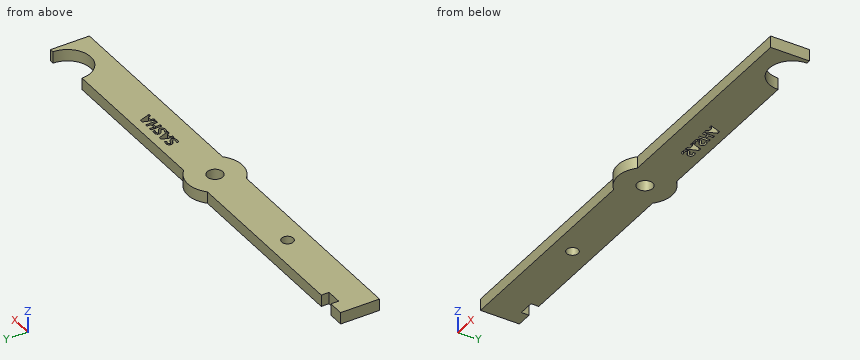
from build123d import *

# Parameters (mm, degrees)
F0_R     = 1.5
F0_R_2   = 2
F1_DEPTH = 3


with BuildPart() as f1:
    # F0 (on Top) → F1 (new body)
    with BuildSketch(Plane.XY):
        with BuildLine():
            Line((-56, 5), (-60, 5))
            Line((-60, 5), (-60, -5))
            Line((-60, -5), (-4.8989794856, -5))
            ThreePointArc((-4.8989794856, -5), (-7, 0), (-4.8989794856, 5))
            Line((-4.8989794856, 5), (-52, 5))
            Line((-52, 5), (-52, 3))
            Line((-52, 3), (-56, 3))
            Line((-56, 3), (-56, 5))
        make_face()
        with Locations((-30, 0)):
            Circle(F0_R, mode=Mode.SUBTRACT)
        with BuildLine():
            ThreePointArc((7, 0), (6.4534043883, -2.7117470016), (4.8989794856, -5))
            Line((4.8989794856, -5), (60, -5))
            Line((60, -5), (60, 5))
            Line((60, 5), (59, 5))
            ThreePointArc((59, 5), (53, -1), (47, 5))
            Line((47, 5), (4.8989794856, 5))
            ThreePointArc((4.8989794856, 5), (6.4534043883, 2.7117470016), (7, 0))
        make_face()
        with BuildLine():
            add(Edge.make_bspline(
                [(16.4754206125, 1.2379939809), (16.6207250703, 1.049862946), (16.6207250703, 0.7763846611)],
                knots=[0, 0, 0, 1, 1, 1], degree=2))
            add(Edge.make_bspline(
                [(16.6207250703, 0.7763846611), (16.6207250703, 0.3976753583), (16.3481644978, 0.1795657195)],
                knots=[0, 0, 0, 1, 1, 1], degree=2))
            add(Edge.make_bspline(
                [(16.3481644978, 0.1795657195), (16.0756039253, -0.0385439193), (15.5904399881, -0.0385439193)],
                knots=[0, 0, 0, 1, 1, 1], degree=2))
            add(Edge.make_bspline(
                [(15.5904399881, -0.0385439193), (15.1425963539, -0.0385439193), (14.798760121, 0.1303151559)],
                knots=[0, 0, 0, 1, 1, 1], degree=2))
            Line((14.798760121, 0.1303151559), (14.798760121, 0.6809425751))
            add(Edge.make_bspline(
                [(14.798760121, 0.6809425751), (15.0814155295, 0.5542982687), (15.2775000716, 0.5029063762)],
                knots=[0, 0, 0, 1, 1, 1], degree=2))
            add(Edge.make_bspline(
                [(15.2775000716, 0.5029063762), (15.4735846136, 0.4515144838), (15.6363256064, 0.4515144838)],
                knots=[0, 0, 0, 1, 1, 1], degree=2))
            add(Edge.make_bspline(
                [(15.6363256064, 0.4515144838), (15.8308806279, 0.4515144838), (15.9351939334, 0.5258491854)],
                knots=[0, 0, 0, 1, 1, 1], degree=2))
            add(Edge.make_bspline(
                [(15.9351939334, 0.5258491854), (16.0395072389, 0.6001838869), (16.0395072389, 0.7476296736)],
                knots=[0, 0, 0, 1, 1, 1], degree=2))
            add(Edge.make_bspline(
                [(16.0395072389, 0.7476296736), (16.0395072389, 0.8296119783), (15.9936216207, 0.8938518439)],
                knots=[0, 0, 0, 1, 1, 1], degree=2))
            add(Edge.make_bspline(
                [(15.9936216207, 0.8938518439), (15.9477360024, 0.9580917094), (15.858717903, 1.0171312049)],
                knots=[0, 0, 0, 1, 1, 1], degree=2))
            add(Edge.make_bspline(
                [(15.858717903, 1.0171312049), (15.7696998035, 1.0761707004), (15.4962215186, 1.2064858563)],
                knots=[0, 0, 0, 1, 1, 1], degree=2))
            add(Edge.make_bspline(
                [(15.4962215186, 1.2064858563), (15.2404856728, 1.3270120803), (15.1123118458, 1.4377493724)],
                knots=[0, 0, 0, 1, 1, 1], degree=2))
            add(Edge.make_bspline(
                [(15.1123118458, 1.4377493724), (14.9841380188, 1.5484866645), (14.9076619883, 1.6959324512)],
                knots=[0, 0, 0, 1, 1, 1], degree=2))
            add(Edge.make_bspline(
                [(14.9076619883, 1.6959324512), (14.8311859579, 1.8433782379), (14.8311859579, 2.0397686841)],
                knots=[0, 0, 0, 1, 1, 1], degree=2))
            add(Edge.make_bspline(
                [(14.8311859579, 2.0397686841), (14.8311859579, 2.4111362879), (15.082639146, 2.6231278443)],
                knots=[0, 0, 0, 1, 1, 1], degree=2))
            add(Edge.make_bspline(
                [(15.082639146, 2.6231278443), (15.3340923341, 2.8351194007), (15.7776533107, 2.8351194007)],
                knots=[0, 0, 0, 1, 1, 1], degree=2))
            add(Edge.make_bspline(
                [(15.7776533107, 2.8351194007), (15.9954570454, 2.8351194007), (16.1933770122, 2.7837275083)],
                knots=[0, 0, 0, 1, 1, 1], degree=2))
            add(Edge.make_bspline(
                [(16.1933770122, 2.7837275083), (16.391296979, 2.7323356158), (16.607265289, 2.6387289545)],
                knots=[0, 0, 0, 1, 1, 1], degree=2))
            Line((16.607265289, 2.6387289545), (16.416381117, 2.1774255389))
            add(Edge.make_bspline(
                [(16.416381117, 2.1774255389), (16.1924592998, 2.2691967754), (16.0462371296, 2.3055993659)],
                knots=[0, 0, 0, 1, 1, 1], degree=2))
            add(Edge.make_bspline(
                [(16.0462371296, 2.3055993659), (15.9000149594, 2.3420019564), (15.7586872551, 2.3420019564)],
                knots=[0, 0, 0, 1, 1, 1], degree=2))
            add(Edge.make_bspline(
                [(15.7586872551, 2.3420019564), (15.5904399881, 2.3420019564), (15.5005041763, 2.2636905012)],
                knots=[0, 0, 0, 1, 1, 1], degree=2))
            add(Edge.make_bspline(
                [(15.5005041763, 2.2636905012), (15.4105683645, 2.185379046), (15.4105683645, 2.0593465479)],
                knots=[0, 0, 0, 1, 1, 1], degree=2))
            add(Edge.make_bspline(
                [(15.4105683645, 2.0593465479), (15.4105683645, 1.9810350927), (15.446970955, 1.9226074054)],
                knots=[0, 0, 0, 1, 1, 1], degree=2))
            add(Edge.make_bspline(
                [(15.446970955, 1.9226074054), (15.4833735455, 1.8641797182), (15.5626027131, 1.8097287845)],
                knots=[0, 0, 0, 1, 1, 1], degree=2))
            add(Edge.make_bspline(
                [(15.5626027131, 1.8097287845), (15.6418318806, 1.7552778508), (15.9379470705, 1.6139501465)],
                knots=[0, 0, 0, 1, 1, 1], degree=2))
            add(Edge.make_bspline(
                [(15.9379470705, 1.6139501465), (16.3301161546, 1.4261250158), (16.4754206125, 1.2379939809)],
                knots=[0, 0, 0, 1, 1, 1], degree=2))
        make_face(mode=Mode.SUBTRACT)
        Polygon((19.4772577596, 0), (18.8385299533, 0), (18.6360214247, 0.665647369), (17.6167488909, 0.665647369), (17.4142403622, 0), (16.7755125559, 0), (17.7623592528, 2.8069762215), (18.4867402132, 2.8069762215), align=None, mode=Mode.SUBTRACT)
        with BuildLine():
            add(Edge.make_bspline(
                [(21.3337898747, 1.2379939809), (21.4790943325, 1.049862946), (21.4790943325, 0.7763846611)],
                knots=[0, 0, 0, 1, 1, 1], degree=2))
            add(Edge.make_bspline(
                [(21.4790943325, 0.7763846611), (21.4790943325, 0.3976753583), (21.20653376, 0.1795657195)],
                knots=[0, 0, 0, 1, 1, 1], degree=2))
            add(Edge.make_bspline(
                [(21.20653376, 0.1795657195), (20.9339731875, -0.0385439193), (20.4488092504, -0.0385439193)],
                knots=[0, 0, 0, 1, 1, 1], degree=2))
            add(Edge.make_bspline(
                [(20.4488092504, -0.0385439193), (20.0009656161, -0.0385439193), (19.6571293832, 0.1303151559)],
                knots=[0, 0, 0, 1, 1, 1], degree=2))
            Line((19.6571293832, 0.1303151559), (19.6571293832, 0.6809425751))
            add(Edge.make_bspline(
                [(19.6571293832, 0.6809425751), (19.9397847917, 0.5542982687), (20.1358693338, 0.5029063762)],
                knots=[0, 0, 0, 1, 1, 1], degree=2))
            add(Edge.make_bspline(
                [(20.1358693338, 0.5029063762), (20.3319538758, 0.4515144838), (20.4946948686, 0.4515144838)],
                knots=[0, 0, 0, 1, 1, 1], degree=2))
            add(Edge.make_bspline(
                [(20.4946948686, 0.4515144838), (20.6892498901, 0.4515144838), (20.7935631956, 0.5258491854)],
                knots=[0, 0, 0, 1, 1, 1], degree=2))
            add(Edge.make_bspline(
                [(20.7935631956, 0.5258491854), (20.8978765011, 0.6001838869), (20.8978765011, 0.7476296736)],
                knots=[0, 0, 0, 1, 1, 1], degree=2))
            add(Edge.make_bspline(
                [(20.8978765011, 0.7476296736), (20.8978765011, 0.8296119783), (20.8519908829, 0.8938518439)],
                knots=[0, 0, 0, 1, 1, 1], degree=2))
            add(Edge.make_bspline(
                [(20.8519908829, 0.8938518439), (20.8061052646, 0.9580917094), (20.7170871652, 1.0171312049)],
                knots=[0, 0, 0, 1, 1, 1], degree=2))
            add(Edge.make_bspline(
                [(20.7170871652, 1.0171312049), (20.6280690657, 1.0761707004), (20.3545907808, 1.2064858563)],
                knots=[0, 0, 0, 1, 1, 1], degree=2))
            add(Edge.make_bspline(
                [(20.3545907808, 1.2064858563), (20.098854935, 1.3270120803), (19.970681108, 1.4377493724)],
                knots=[0, 0, 0, 1, 1, 1], degree=2))
            add(Edge.make_bspline(
                [(19.970681108, 1.4377493724), (19.842507281, 1.5484866645), (19.7660312505, 1.6959324512)],
                knots=[0, 0, 0, 1, 1, 1], degree=2))
            add(Edge.make_bspline(
                [(19.7660312505, 1.6959324512), (19.6895552201, 1.8433782379), (19.6895552201, 2.0397686841)],
                knots=[0, 0, 0, 1, 1, 1], degree=2))
            add(Edge.make_bspline(
                [(19.6895552201, 2.0397686841), (19.6895552201, 2.4111362879), (19.9410084082, 2.6231278443)],
                knots=[0, 0, 0, 1, 1, 1], degree=2))
            add(Edge.make_bspline(
                [(19.9410084082, 2.6231278443), (20.1924615963, 2.8351194007), (20.6360225729, 2.8351194007)],
                knots=[0, 0, 0, 1, 1, 1], degree=2))
            add(Edge.make_bspline(
                [(20.6360225729, 2.8351194007), (20.8538263076, 2.8351194007), (21.0517462744, 2.7837275083)],
                knots=[0, 0, 0, 1, 1, 1], degree=2))
            add(Edge.make_bspline(
                [(21.0517462744, 2.7837275083), (21.2496662412, 2.7323356158), (21.4656345512, 2.6387289545)],
                knots=[0, 0, 0, 1, 1, 1], degree=2))
            Line((21.4656345512, 2.6387289545), (21.2747503792, 2.1774255389))
            add(Edge.make_bspline(
                [(21.2747503792, 2.1774255389), (21.050828562, 2.2691967754), (20.9046063918, 2.3055993659)],
                knots=[0, 0, 0, 1, 1, 1], degree=2))
            add(Edge.make_bspline(
                [(20.9046063918, 2.3055993659), (20.7583842216, 2.3420019564), (20.6170565173, 2.3420019564)],
                knots=[0, 0, 0, 1, 1, 1], degree=2))
            add(Edge.make_bspline(
                [(20.6170565173, 2.3420019564), (20.4488092504, 2.3420019564), (20.3588734386, 2.2636905012)],
                knots=[0, 0, 0, 1, 1, 1], degree=2))
            add(Edge.make_bspline(
                [(20.3588734386, 2.2636905012), (20.2689376267, 2.185379046), (20.2689376267, 2.0593465479)],
                knots=[0, 0, 0, 1, 1, 1], degree=2))
            add(Edge.make_bspline(
                [(20.2689376267, 2.0593465479), (20.2689376267, 1.9810350927), (20.3053402172, 1.9226074054)],
                knots=[0, 0, 0, 1, 1, 1], degree=2))
            add(Edge.make_bspline(
                [(20.3053402172, 1.9226074054), (20.3417428077, 1.8641797182), (20.4209719753, 1.8097287845)],
                knots=[0, 0, 0, 1, 1, 1], degree=2))
            add(Edge.make_bspline(
                [(20.4209719753, 1.8097287845), (20.5002011428, 1.7552778508), (20.7963163327, 1.6139501465)],
                knots=[0, 0, 0, 1, 1, 1], degree=2))
            add(Edge.make_bspline(
                [(20.7963163327, 1.6139501465), (21.1884854168, 1.4261250158), (21.3337898747, 1.2379939809)],
                knots=[0, 0, 0, 1, 1, 1], degree=2))
        make_face(mode=Mode.SUBTRACT)
        Polygon((24.2762816222, 2.7953518649), (24.2762816222, 0), (23.6852748589, 0), (23.6852748589, 1.2064858563), (22.5785137462, 1.2064858563), (22.5785137462, 0), (21.9856715582, 0), (21.9856715582, 2.7953518649), (22.5785137462, 2.7953518649), (22.5785137462, 1.6996033006), (23.6852748589, 1.6996033006), (23.6852748589, 2.7953518649), align=None, mode=Mode.SUBTRACT)
        Polygon((27.3316519906, 0), (26.6929241843, 0), (26.4904156556, 0.665647369), (25.4711431219, 0.665647369), (25.2686345932, 0), (24.6299067869, 0), (25.6167534838, 2.8069762215), (26.3411344442, 2.8069762215), align=None, mode=Mode.SUBTRACT)
        with BuildLine():
            ThreePointArc((-4.8989794856, 5), (-7, 0), (-4.8989794856, -5))
            Line((-4.8989794856, -5), (4.8989794856, -5))
            ThreePointArc((4.8989794856, -5), (6.4534043883, -2.7117470016), (7, 0))
            ThreePointArc((7, 0), (6.4534043883, 2.7117470016), (4.8989794856, 5))
            Line((4.8989794856, 5), (-4.8989794856, 5))
        make_face()
        Circle(F0_R_2, mode=Mode.SUBTRACT)
        with BuildLine():
            ThreePointArc((4.8989794856, 5), (0, 7), (-4.8989794856, 5))
            Line((-4.8989794856, 5), (4.8989794856, 5))
        make_face()
        with BuildLine():
            Line((4.8989794856, -5), (-4.8989794856, -5))
            ThreePointArc((-4.8989794856, -5), (0, -7), (4.8989794856, -5))
        make_face()
    extrude(amount=F1_DEPTH)


solid = f1.part
For this review, take the finished solid that the model builds, in its own axes (mm). Round coordinates to 2 decimals unless told otherwise and drop trailing zeros. Loops run counter-clockwise (first coordinate to the right, second up) from the corner with the lowest first, then second, coordinate; pieces in that order, holes last. Notation, with made-up numbers: (41.5, 67.5) - (47.5, 67.5) arc R32 ccw to (47.5, 104.5) - close; hole circle Ø10 at (81, -28). An arc over 180 degrees is marked (long way). Use one line per item in the form item = value.
Item 1: Clearance check with flat-ended pins moving along their axes: P1, Ø0.6, axis at x = 23, z = 2, coming from the -Y side; P2, Ø1, axis at x = -46, z = 1.5, coming from the +Y side. State where each tip first meets the part, or that it passes through.
Answers:
P1 = -5
P2 = 5
Item 2: Consider section A-A on x = 0. Write out the cut boundary in (y, z).
Answers:
outline = (-7, 0) - (-2, 0) - (-2, 3) - (-7, 3) - close; (2, 0) - (7, 0) - (7, 3) - (2, 3) - close
Item 3: Consider section B-B on x = -30. Write out the cut boundary in (y, z).
Answers:
outline = (-5, 0) - (-1.5, 0) - (-1.5, 3) - (-5, 3) - close; (1.5, 0) - (5, 0) - (5, 3) - (1.5, 3) - close
Item 4: For line 1 (Y direction, x = -30, z = 2); line 2 (X direction, y = 3.5, z = 0.8); line 3 (Y direction, x = -52.5, z = 2.35), list the stretches that pass through material, from the lowest coordinate up.
Answers:
line_1 = -5 to -1.5, 1.5 to 5
line_2 = -60 to -56, -52 to 47.19, 58.81 to 60
line_3 = -5 to 3
Item 5: Consider section C-C on z = 1.65. State how many separate pieces and enclosed holes the cut face has, then the cut area to 3 significant figures.
Answers:
separate_pieces = 1
enclosed_holes = 7
area = 1,130 mm^2
Item 6: Consider section D-D on x = 38. Write out the cut boundary in (y, z).
Answers:
outline = (-5, 0) - (5, 0) - (5, 3) - (-5, 3) - close
